Autodesk Inventor part; units mm, degrees
ref_plane "YZ Plane" through (0, 0, 0) normal (1, 0, 0) x (0, 1, 0)
ref_plane "XZ Plane" through (0, 0, 0) normal (0, 1, 0) x (-1, 0, 0)
ref_plane "XY Plane" through (0, 0, 0) normal (0, 0, 1) x (1, 0, 0)
sketch "Sketch1" plane through (0, 0, 0) normal (0, 1, 0) x (-1, 0, 0)
  line L0 (19.3231, -122.2306) -> (-6.0769, -122.2306)
  circle A0 centre (32.0231, -7.9306) radius 3.175
  circle A1 centre (6.6231, -109.5306) radius 3.175
  line L1 (19.3231, -122.2306) -> (44.7231, -20.6306)
  line L2 (44.7231, -20.6306) -> (44.7231, 4.7694)
  line L3 (-6.0769, -122.2306) -> (6.6231, 4.7694)
  line L4 (6.6231, 4.7694) -> (44.7231, 4.7694)
  dimension "d0" = 25.4
  dimension "d2" = 6.35
  dimension "d3" = 6.35
  dimension "d6" = 12.7
  dimension "d10" = 25.4
  dimension "d12" = 12.7
  dimension "d13" = 38.1
  dimension "d14" = 12.7
  dimension "d15" = 12.7
  dimension "d16" = 50.8
  dimension "d17" = 127
extrude "Extrusion1" add sketch "Sketch1" along normal blind 3.175
properties part number "15102898-16-P-0213" material "Aluminum 6061"
Can you work these out from the model? Positions are in its coordinate system, mm. Coordinates: 2 decimals unless noted, no trailing zeros. Loops run counter-clockwise (first coordinate to the right, second up) from the corner with the lowest first, then second, coordinate; pieces in that order, holes last. Notation, with made-up numbers: (-28, -32) - (-17, -32) arc R31 cw to (-17, -5) - close; hole circle Ø4 at (35, 60.5). An arc over 180 degrees is marked (long way). Answer as CSV lines item,"result". Start each with the question number.
1) Suppose I cut it at D-D (x = -25.5). Please give me the cut outline in (y, z) (3 decimals), plus the area to 3 significant figures.
2) I need wall thicknesses on line 1 (X direction, y = 3.05, z = -110.5); line 2 (X direction, y = 0.55, z = -7.5); line 3 (X direction, y = 2.2, z = -94.5). Which ranges of each line are inside material? Lowest first, please. Write a range as from..to.
3) Suppose I cut it at A-A (x = -33). Please give me the cut outline in (y, z) (3 decimals).
4) For pin 1 (10 mm diameter, centred on x = -32.02, z = -7.93, fed in from -Y); pin 2 (5.5 mm diameter, centred on x = -6.62, z = -109.53, fed in from +Y), each with a flat end and sliding along its axis, tell me the tip position at first contact or that it passes through.
5) Thinking about a two-plate mould opening in Z: for faces 1 (the flat face through (-25, 2, 4.769)), 2 (the flat face through (-31.845, 1.565, -72.142)), 3 (the cylindrical face through (-6.21, 1.57, -112.68)), 4 (the flat face through (-19, 0, -58)), which applies, pulls with the +Z half, pulls with the -Z half, needs draft (parallel to the pull), parting line crosses it, or undercut?
6) Suppose I cut it at C-C (z = -12.5). Please give me the cut outline in (x, y) (3 decimals).
7) Suppose I cut it at B-B (y = 1.6). Please give me the cut outline in (x, z) (3 decimals).
Check result:
1,outline,"(0, -97.523) - (3.175, -97.523) - (3.175, 4.769) - (0, 4.769) - close"
1,area,"325 mm²"
2,line 1,"x = -22.26..-9.65, -3.6..4.9"
2,line 2,"x = -44.72..-35.17, -28.88..-5.4"
2,line 3,"x = -26.26..3.3"
3,outline,"(0, -67.523) - (3.175, -67.523) - (3.175, -10.952) - (0, -10.952) - close; (0, -4.91) - (3.175, -4.91) - (3.175, 4.769) - (0, 4.769) - close"
4,pin 1,"stops at y = 0"
4,pin 2,"passes through"
5,face 1,"pulls with the +Z half"
5,face 2,"pulls with the -Z half"
5,face 3,"undercut"
5,face 4,"needs draft"
6,outline,"(-44.723, 0) - (-4.896, 0) - (-4.896, 3.175) - (-44.723, 3.175) - close"
7,outline,"(-44.723, -20.631) - (-19.323, -122.231) - (6.077, -122.231) - (-6.623, 4.769) - (-44.723, 4.769) - close; hole circle Ø6.35 at (-32.023, -7.931); hole circle Ø6.35 at (-6.623, -109.531)"
